from build123d import *

# Parameters (mm, degrees)
SKETCH1_R           = 38.1
BOSS_EXTRUDE1_DEPTH = 76.2
SHELL2_T            = 3.175
SKETCH2_W           = 3
SKETCH2_H           = 75
SKETCH2_H_2         = 48.033738144
SKETCH2_H_3         = 61.308726948
SKETCH2_H_4         = 69.24998195
SKETCH2_H_5         = 73.60461942
BOSS_EXTRUDE2_DEPTH = 7
SCALE1_SCALE        = 0.615384615


with BuildPart() as part:
    # Sketch1 → Boss-Extrude1 (new body)
    with BuildSketch(Plane(origin=(0, 0, 0), x_dir=(1, 0, 0), z_dir=(0, 1, 0))):
        with Locations(Location((0, 0, 0), (0, 0, 90))):
            Circle(SKETCH1_R)
    extrude(amount=BOSS_EXTRUDE1_DEPTH)

    # Shell2
    shell2_openings = [part.faces().sort_by_distance(p)[0] for p in [
        (0, 76.2, 0),
    ]]
    offset(amount=SHELL2_T, openings=shell2_openings, kind=Kind.INTERSECTION)

    # Sketch2 → Boss-Extrude2 (add)
    with BuildSketch(Plane.XZ.offset(3.175)):
        Rectangle(SKETCH2_W, SKETCH2_H)
        Polygon((-34.5, -10.5), (-34.5, 0), (-34.5, 10.5), (-37.5, 10.5), (-37.5, -10.5), align=None)
        with Locations((-28.8, 0)):
            Rectangle(SKETCH2_W, SKETCH2_H_2)
        with Locations((-21.6, 0)):
            Rectangle(SKETCH2_W, SKETCH2_H_3)
        with Locations((-14.4, 0)):
            Rectangle(SKETCH2_W, SKETCH2_H_4)
        with Locations((-7.2, 0)):
            Rectangle(SKETCH2_W, SKETCH2_H_5)
        Polygon((8.7, -36.80230971), (8.7, 0), (8.7, 36.80230971), (5.7, 36.80230971), (5.7, -36.80230971), align=None)
        with Locations((14.4, 0)):
            Rectangle(SKETCH2_W, SKETCH2_H_4)
        with Locations((21.6, 0)):
            Rectangle(SKETCH2_W, SKETCH2_H_3)
        with Locations((28.8, 0)):
            Rectangle(SKETCH2_W, SKETCH2_H_2)
        Polygon((37.5, -10.5), (37.5, 10.5), (34.5, 10.5), (34.5, 0), (34.5, -10.5), align=None)
    extrude(amount=BOSS_EXTRUDE2_DEPTH)


with BuildPart() as part_1:
    # Scale1: scaled about (0, 24.172158943, 0)
    add(part.part.scale(SCALE1_SCALE).moved(Location((0, 9.296984209, 0))))


solid = part_1.part
Model file for the job. Use its own axes, mm. A direction names the side the tool comes from. Give positions to 0.01 mm unless a question says otherwise; leave off trailing zeros. Loops run counter-clockwise (first coordinate to the right, second up) from the corner with the lowest first, then second, coordinate; pieces in that order, holes last.
1) Saw through at A-A (x = 0). Write the cut outline in (y, z).
2) Wall check: line 1 (X direction, y = 7, z = -21); line 2 (X direction, y = 40, z = 0); line 3 (Y direction, x = -6.5, z = 2.5). Give the ranges that are in metal, low to high.
3) Saw through at D-D (x = 7). Write the cut outline in (y, z).
4) Saw through at C-C (x = -11). Write the cut outline in (y, z).
5) Pull direction X, two halves, no side cores. Call faces 5 (the flat face through (-22, 5, 6.462)), 6 (the flat face through (-12.369, 5, 0)): +X half, -X half, draft (parallel to the pull), parting line (faces both ways), or undercut.
6) Saw through at B-B (y = 51.5). Write the cut outline in (x, z), plus the area to 3 significant figures.
7) Tool access for faces 1 (the flat face through (0, 5, 23.077)), 2 (the flat face through (18, 5, 14.78)), 3 (the flat face through (-9, 5, 21.308)), 4 (the flat face through (-21.231, 5, 0)): list every direction of +Z, -Z, +X, -X, +Y, -Y with a clear straight run to the whole face (end or side of a thin tool).
8) Flat gauge pins, fed straight in: pin 1 Ø2 at (x, y) = (22, 6) entering from +Z; pin 2 Ø0.9 at (x, y) = (13, 6) entering from -Z; pin 3 Ø1.3 at (y, z) = (4.5, 8) entering from +X; pin 4 Ø5 at (x, z) = (-19, 3.5) entering from -Y. Where does each tip first touch, or does it go through?
Answer block:
1. outline: (3.04, -23.08) - (7.34, -23.08) - (7.34, -25.4) - (56.19, -25.4) - (56.19, -23.45) - (9.3, -23.45) - (9.3, 23.45) - (56.19, 23.45) - (56.19, 25.4) - (7.34, 25.4) - (7.34, 23.08) - (3.04, 23.08) - close
2. line 1: x = -9.78 to -7.94, -5.35 to -3.51, -0.92 to 0.92, 3.51 to 5.35, 7.94 to 9.78
2. line 2: x = -25.4 to -23.45, 23.45 to 25.4
2. line 3: y = 7.34 to 9.3
3. outline: (7.34, -24.42) - (56.19, -24.42) - (56.19, -22.38) - (9.3, -22.38) - (9.3, 22.38) - (56.19, 22.38) - (56.19, 24.42) - (7.34, 24.42) - close
4. outline: (7.34, -22.89) - (56.19, -22.89) - (56.19, -20.71) - (9.3, -20.71) - (9.3, 20.71) - (56.19, 20.71) - (56.19, 22.89) - (7.34, 22.89) - close
5. face 5: draft
5. face 6: undercut
6. outline: circle Ø50.8 at (0, 0); hole circle Ø46.89 at (0, 0)
6. area: 300 mm2
7. face 1: +Z, +X, -X, -Y
7. face 2: +Z, +X, -Y
7. face 3: +Z, -X, -Y
7. face 4: +Z, -Z, -Y
8. pin 1: stops at z = 6.46
8. pin 2: stops at z = -18.86
8. pin 3: stops at x = 18.65
8. pin 4: stops at y = 3.04
